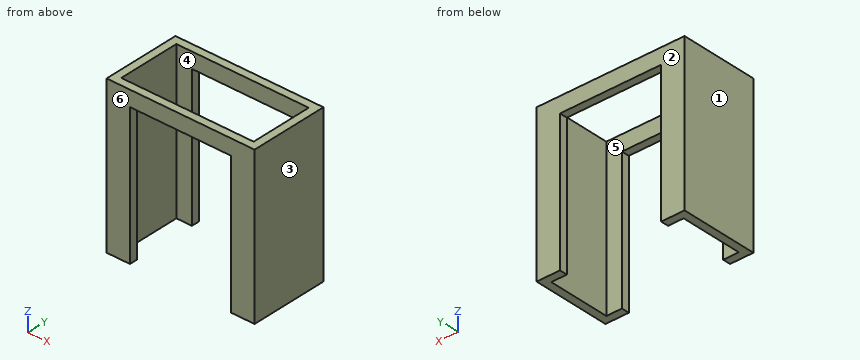
from build123d import *

# Parameters (mm, degrees)
SKETCH1_W                = 19
SKETCH1_H                = 10
BOSS_EXTRUDE1_DEPTH      = 10
BOSS_EXTRUDE1_DEPTH_BACK = 10
SKETCH2_W                = 17
SKETCH2_H                = 8
CUT_EXTRUDE1_DEPTH       = 20
SKETCH3_W                = 13
SKETCH3_H                = 10.51996768
CUT_EXTRUDE3_DEPTH       = 8
CUT_EXTRUDE3_DEPTH_BACK  = 10


with BuildPart() as part:
    # Sketch1 → Boss-Extrude1 (new body, two sides)
    with BuildSketch(Plane.XY) as boss_extrude1_sk:
        with Locations((-0.130136986, 2.22260274)):
            Rectangle(SKETCH1_W, SKETCH1_H)
    extrude(amount=BOSS_EXTRUDE1_DEPTH)
    extrude(boss_extrude1_sk.sketch, amount=-BOSS_EXTRUDE1_DEPTH_BACK)

    # Sketch2 → Cut-Extrude1 (cut)
    with BuildSketch(Plane.XY.offset(10)):
        with Locations((-0.130136986, 2.22260274)):
            Rectangle(SKETCH2_W, SKETCH2_H)
    extrude(amount=-CUT_EXTRUDE1_DEPTH, mode=Mode.SUBTRACT)

    # Sketch3 → Cut-Extrude3 (cut, two sides)
    with BuildSketch(Plane.XY) as cut_extrude3_sk:
        with Locations((-0.130136986, 2.34516547)):
            Rectangle(SKETCH3_W, SKETCH3_H)
    extrude(amount=CUT_EXTRUDE3_DEPTH, mode=Mode.SUBTRACT)
    extrude(cut_extrude3_sk.sketch, amount=-CUT_EXTRUDE3_DEPTH_BACK, mode=Mode.SUBTRACT)


solid = part.part
Here's how the part is built. I have some questions about the finished solid (model axes, mm). Face numbers are marked on the shaded views. A direction names the side the tool comes from. Give positions to 0.01 mm unless a question says otherwise; leave off trailing zeros. Loops run counter-clockwise (first coordinate to the right, second up) from the corner with the lowest first, then second, coordinate; pieces in that order, holes last. Notation, with made-up numbers: (53.25, 46.5) -> (93.25, 46.5) arc R12 ccw to (93.25, 59.5) -> close; hole circle Ø2 at (32.25, -19.75). An arc over 180 degrees is marked (long way). Answer as a JSON object with one key per item and string values. Group by question number.
Item 1: Thinking about a two-plate mould opening in X: for the marked faces 1, 2, 3 and 4, which applies, pulls with the +X half, pulls with the -X half, needs draft (parallel to the pull), parting line crosses it, or undercut?
Item 2: Imagine slicing it at D-D on y = 6.75. Write out the boundary of the cut face in (x, z).
Item 3: I need wall thicknesses on L1, parallel to Y at x = 6.75, z = -2; L2, parallel to X at y = 6, z = 2. Which ranges of each line are inside material? Lowest first, please.
Item 4: Imagine slicing it at A-A on x = 0. Write out the boundary of the cut face in (y, z).
Item 5: Will this pin go through, and if not, where does the flat tip stop? pin 1 (0.8 mm diameter, centred on x = -1, y = 7, fed in from -Z).
Item 6: Imagine slicing it at B-B on y = 4.25. Write out the boundary of the cut face in (x, z), then the cut area to 3 significant figures.
Item 7: On a 3-axis mill with a long thin cutter (end or side, diameter ignored), from which of +Z, -Z, +X, -X, +Y, -Y can I reach the whole of each face in a straight line? I mean the marked faces 5 and 6. Say none if no direction works.
Item 8: Imagine slicing it at C-C on z = -4.5. Write out the boundary of the cut face in (x, y).
Answer list:
{
 "1": {"face 1": "pulls with the -X half", "face 2": "needs draft", "face 3": "pulls with the +X half", "face 4": "undercut"},
 "2": {"outline": "(-9.63, -10) -> (-6.63, -10) -> (-6.63, 8) -> (6.37, 8) -> (6.37, -10) -> (9.37, -10) -> (9.37, 10) -> (-9.63, 10) -> close"},
 "3": {"L1": "y = -2.78 to -1.78, 6.22 to 7.22", "L2": "x = -9.63 to -8.63, 8.37 to 9.37"},
 "4": {"outline": "(-2.78, 8) -> (-1.78, 8) -> (-1.78, 10) -> (-2.78, 10) -> close; (6.22, 8) -> (7.22, 8) -> (7.22, 10) -> (6.22, 10) -> close"},
 "5": {"pin 1": "stops at z = 8"},
 "6": {"outline": "(-9.63, -10) -> (-8.63, -10) -> (-8.63, 10) -> (-9.63, 10) -> close; (8.37, -10) -> (9.37, -10) -> (9.37, 10) -> (8.37, 10) -> close", "area": "40.0 mm2"},
 "7": {"face 5": "+Z, -Z", "face 6": "+Z, -Z, +X, -X, -Y"},
 "8": {"outline": "(-9.63, -2.78) -> (-6.63, -2.78) -> (-6.63, -1.78) -> (-8.63, -1.78) -> (-8.63, 6.22) -> (-6.63, 6.22) -> (-6.63, 7.22) -> (-9.63, 7.22) -> close; (6.37, -2.78) -> (9.37, -2.78) -> (9.37, 7.22) -> (6.37, 7.22) -> (6.37, 6.22) -> (8.37, 6.22) -> (8.37, -1.78) -> (6.37, -1.78) -> close"}
}
